```python
from build123d import *

# Parameters (mm, degrees)
SKETCH1_W                    = 67
SKETCH1_H                    = 67
BOSS_EXTRUDE1_DEPTH          = 67
SKETCH2_W                    = 57
SKETCH2_H                    = 57
CUT_EXTRUDE1_DEPTH           = 47
CUT_EXTRUDE2_REACH           = 102.5
SKETCH3_R                    = 10.75
CUT_EXTRUDE3_REACH           = 102.5
SKETCH4_R                    = 10.75
F_5_0_5_DIAMETER_HOLE1_D     = 5
F_5_0_5_DIAMETER_HOLE1_DEPTH = 5
F_5_0_5_DIAMETER_HOLE1_TIP   = 1.502151548
FILLET1_R                    = 5
CHAMFER1_SIZE                = 3.04
CUT_EXTRUDE4_REACH           = 102.5
CUT_EXTRUDE5_DEPTH           = 101.5
SKETCH9_R                    = 1.5
CUT_EXTRUDE6_DEPTH           = 10
SKETCH10_R                   = 1.5
CUT_EXTRUDE7_DEPTH           = 10


with BuildPart() as part:
    # Sketch1 → Boss-Extrude1 (new body)
    with BuildSketch(Plane(origin=(0, 0, 0), x_dir=(1, 0, 0), z_dir=(0, 1, 0))):
        Rectangle(SKETCH1_W, SKETCH1_H)
    extrude(amount=BOSS_EXTRUDE1_DEPTH)

    # Sketch2 → Cut-Extrude1 (cut)
    with BuildSketch(Plane(origin=(0, 67, 0), x_dir=(1, 0, 0), z_dir=(0, 1, 0))):
        with Locations((5, -5)):
            Rectangle(SKETCH2_W, SKETCH2_H)
    extrude(amount=-CUT_EXTRUDE1_DEPTH, mode=Mode.SUBTRACT)

    # Sketch3 → Cut-Extrude2 (cut, up to next)
    with BuildSketch(Plane.ZY.offset(33.5), mode=Mode.PRIVATE) as cut_extrude2_sk1:
        with Locations((11.5, 50)):
            Circle(SKETCH3_R)
    cut_extrude2_tool1 = extrude(cut_extrude2_sk1.sketch, amount=-CUT_EXTRUDE2_REACH, mode=Mode.PRIVATE) & part.part
    add(cut_extrude2_tool1.solids().sort_by_distance((-33.5, 50, 11.5))[0], mode=Mode.SUBTRACT)

    # Sketch4 → Cut-Extrude3 (cut, up to next)
    with BuildSketch(Plane(origin=(0, 0, -33.5), x_dir=(-1, 0, 0), z_dir=(0, 0, -1)), mode=Mode.PRIVATE) as cut_extrude3_sk1:
        with Locations((-11.5, 50)):
            Circle(SKETCH4_R)
    cut_extrude3_tool1 = extrude(cut_extrude3_sk1.sketch, amount=-CUT_EXTRUDE3_REACH, mode=Mode.PRIVATE) & part.part
    add(cut_extrude3_tool1.solids().sort_by_distance((11.5, 50, -33.5))[0], mode=Mode.SUBTRACT)

    # Ø5.0 (5) Diameter Hole1
    with Locations(Plane(origin=(0, 20, 0), x_dir=(-1, 0, 0), z_dir=(0, 1, 0))):
        with Locations((16, 11.5), (-11.5, -16)):
            Hole(F_5_0_5_DIAMETER_HOLE1_D / 2, depth=F_5_0_5_DIAMETER_HOLE1_DEPTH)
            with Locations((0, 0, -(F_5_0_5_DIAMETER_HOLE1_DEPTH + F_5_0_5_DIAMETER_HOLE1_TIP / 2))):  # 118° drill point
                Cone(0, F_5_0_5_DIAMETER_HOLE1_D / 2, F_5_0_5_DIAMETER_HOLE1_TIP, mode=Mode.SUBTRACT)

    # Fillet1
    fillet1_edges = [part.edges().sort_by_distance(p)[0] for p in [
        (-23.5, 43.5, -23.5),
    ]]
    fillet(fillet1_edges, radius=FILLET1_R)

    # Chamfer1
    chamfer1_edges = [part.edges().sort_by_distance(p)[0] for p in [
        (-33.5, 50, 0.75),
        (22.25, 50, -33.5),
    ]]
    chamfer(chamfer1_edges, length=CHAMFER1_SIZE)

    # Sketch7 → Cut-Extrude4 (cut, up to next)
    with BuildSketch(Plane(origin=(33.5, 0, 0), x_dir=(0, 0, -1), z_dir=(1, 0, 0)), mode=Mode.PRIVATE) as cut_extrude4_sk1:
        Polygon((-2.4, 9.5), (-20.6, 9.5), (-16.84722325, 3), (-21, 3), (-21, 0), (-2, 0), (-2, 3), (-6.15277675, 3), align=None)
    cut_extrude4_tool1 = extrude(cut_extrude4_sk1.sketch, amount=-CUT_EXTRUDE4_REACH, mode=Mode.PRIVATE) & part.part
    add(cut_extrude4_tool1.solids().sort_by_distance((33.5, 4.630961, 11.5))[0], mode=Mode.SUBTRACT)

    # Sketch8 → Cut-Extrude5 (cut, through all)
    with BuildSketch(Plane.XY.offset(33.5)):
        Polygon((2.4, 9.5), (20.6, 9.5), (16.84722325, 3), (21, 3), (21, 0), (2, 0), (2, 3), (6.15277675, 3), align=None)
    extrude(amount=-CUT_EXTRUDE5_DEPTH, mode=Mode.SUBTRACT)

    # Sketch9 → Cut-Extrude6 (cut)
    with BuildSketch(Plane.ZY.offset(33.5)):
        with Locations((-1.490381057, 57.5)):
            Circle(SKETCH9_R)
        with Locations((24.490381057, 57.5)):
            Circle(SKETCH9_R)
        with Locations((11.5, 35)):
            Circle(SKETCH9_R)
    extrude(amount=-CUT_EXTRUDE6_DEPTH, mode=Mode.SUBTRACT)

    # Sketch10 → Cut-Extrude7 (cut)
    with BuildSketch(Plane(origin=(0, 0, -33.5), x_dir=(-1, 0, 0), z_dir=(0, 0, -1))):
        with Locations((1.490381057, 57.5)):
            Circle(SKETCH10_R)
        with Locations((-24.490381057, 57.5)):
            Circle(SKETCH10_R)
        with Locations((-11.5, 35)):
            Circle(SKETCH10_R)
    extrude(amount=-CUT_EXTRUDE7_DEPTH, mode=Mode.SUBTRACT)


solid = part.part
```
For this review, take the finished solid that the model builds, in its own axes (mm). A direction names the side the tool comes from. Coordinates: 2 decimals unless noted, no trailing zeros. Write each loop counter-clockwise with the first axis right and the second up, starting at its lowest first coordinate (ties: lowest second). Pieces come first, ordered by that corner, then holes. Notation, with made-up numbers: (76.5, -19.75) -> (113.5, -19.75) arc R17 ccw to (113.5, -15.75) -> close; hole circle Ø4 at (-12, 58). An arc over 180 degrees is marked (long way). Put each result on its own line as item: value.
Q1. Take a section at C-C, the plane y = 27. State the section outline as (x, z) points, then the cut area to 3 significant figures.
From the geometry:
outline: (-33.5, -33.5) -> (33.5, -33.5) -> (33.5, -23.5) -> (-18.5, -23.5) arc R5 cw to (-23.5, -18.5) -> (-23.5, 33.5) -> (-33.5, 33.5) -> close
area: 1,250 mm2
Q2. Clearance check with flat-ended pins moving along their axes: pin 1 Ø4 at (x, z) = (11.5, -16) entering from -Y; pin 2 Ø1 at (x, z) = (15, -1) entering from +Y; pin 3 Ø1 at (y, z) = (29, -1) entering from +X. State where each tip first meets the part, or that it passes through.
From the geometry:
pin 1: stops at y = 9.5
pin 2: stops at y = 20
pin 3: stops at x = -23.5
Q3. Take a section at B-B, the plane z = -4. State the section outline as (x, y) points.
From the geometry:
outline: (-33.5, 0) -> (2, 0) -> (2, 3) -> (6.15, 3) -> (2.4, 9.5) -> (20.6, 9.5) -> (16.85, 3) -> (21, 3) -> (21, 0) -> (33.5, 0) -> (33.5, 20) -> (-23.5, 20) -> (-23.5, 67) -> (-33.5, 67) -> close
Q4. Take a section at D-D, the plane y = 35. State the section outline as (x, z) points, then the cut area to 3 significant figures.
From the geometry:
outline: (-33.5, -33.5) -> (10, -33.5) -> (10, -23.5) -> (-18.5, -23.5) arc R5 cw to (-23.5, -18.5) -> (-23.5, 10) -> (-33.5, 10) -> close; (-33.5, 13) -> (-23.5, 13) -> (-23.5, 33.5) -> (-33.5, 33.5) -> close; (13, -33.5) -> (33.5, -33.5) -> (33.5, -23.5) -> (13, -23.5) -> close
area: 1,190 mm2
Q5. Take a section at A-A, the plane y = 50. State the section outline as (x, z) points, then the cut area to 3 significant figures.
From the geometry:
outline: (-33.5, -33.5) -> (-2.29, -33.5) -> (0.75, -30.46) -> (0.75, -23.5) -> (-18.5, -23.5) arc R5 cw to (-23.5, -18.5) -> (-23.5, 0.75) -> (-30.46, 0.75) -> (-33.5, -2.29) -> close; (-33.5, 25.29) -> (-30.46, 22.25) -> (-23.5, 22.25) -> (-23.5, 33.5) -> (-33.5, 33.5) -> close; (22.25, -30.46) -> (25.29, -33.5) -> (33.5, -33.5) -> (33.5, -23.5) -> (22.25, -23.5) -> close
area: 797 mm2
Q6. Tool access review of faces 1 (the flat face through (7, 39, -23.5)), 2 (the flat face through (21, 2, 27)), 3 (the flat face through (-13.396, 6.296, 18.75)), 4 (the flat face through (-16, 1, 2)): name each direction out of +Z, -Z, +X, -X, +Y, -Y from which nothing blocks a thin tool from reaching the whole face with its end or side.
From the geometry:
face 1: +Z, +X, +Y
face 2: +Z, -Z, -Y
face 3: +X, -X
face 4: +X, -X, -Y
Q7. The part is to be moulded in two halves that separate along Y. For faces 5 (the flat face through (-16, 0, -16)), 6 (the flat face through (-33.5, 33, 0)), 7 (the flat face through (4.303, 6.204, 25.29)), say which applies: +Y half, -Y half, draft (parallel to the pull), parting line (faces both ways), or undercut.
From the geometry:
face 5: -Y half
face 6: draft
face 7: undercut
Q8. Wall thickness on L1, parallel to Z at x = -26, y = 57; L2, parallel to Z at x = -16, y = 18; L3, parallel to Y at x = -26, z = 3: over which ranges is each line inside the solid? List them lowest first.
From the geometry:
L1: z = -33.5 to -2.9, -0.08 to 3.34, 19.66 to 23.08, 25.9 to 33.5
L2: z = -33.5 to 9, 14 to 33.5
L3: y = 3 to 8.46, 9.5 to 43.42, 56.58 to 67
